from build123d import *

# Parameters (mm, degrees)
SKETCH2_R               = 21
SKETCH2_R_2             = 10.5
CUT_EXTRUDE1_DEPTH      = 11
CUT_EXTRUDE1_DEPTH_BACK = 12
SKETCH2_5_R             = 10.5
CUT_EXTRUDE2_DEPTH      = 12
CHAMFER1_SIZE           = 0.5


with BuildPart() as part:
    # Sketch1 → Revolve1 (revolve)
    with BuildSketch(Plane.XY):
        with BuildLine():
            Line((0, 10), (0, -11))
            Line((0, -11), (-21, -11))
            ThreePointArc((-21, -11), (-14.849242405, 3.849242405), (0, 10))
        make_face()
    revolve(axis=Axis((0, 10, 0), (0, -1, 0)))

    # Sketch2 → Cut-Extrude1 (cut, two sides)
    with BuildSketch(Plane(origin=(0, 0, 0), x_dir=(1, 0, 0), z_dir=(0, 1, 0))) as cut_extrude1_sk:
        Circle(SKETCH2_R)
        Circle(SKETCH2_R_2, mode=Mode.SUBTRACT)
    extrude(amount=CUT_EXTRUDE1_DEPTH, mode=Mode.SUBTRACT)
    extrude(cut_extrude1_sk.sketch, amount=-CUT_EXTRUDE1_DEPTH_BACK, mode=Mode.SUBTRACT)

    # Sketch2<5> → Cut-Extrude2 (cut, through all)
    with BuildSketch(Plane(origin=(0, 0, 0), x_dir=(1, 0, 0), z_dir=(0, 1, 0))):
        Circle(SKETCH2_5_R)
    extrude(amount=-CUT_EXTRUDE2_DEPTH, mode=Mode.SUBTRACT)

    # Chamfer1
    chamfer1_edges = [part.edges().sort_by_distance(p)[0] for p in [
        (-10.5, 0, 0),
    ]]
    chamfer(chamfer1_edges, length=CHAMFER1_SIZE)


solid = part.part
Read the model definition and answer for the solid it produces. Units are mm, in the model's axes. Coordinates: 2 decimals unless noted, no trailing zeros. Loops run counter-clockwise (first coordinate to the right, second up) from the corner with the lowest first, then second, coordinate; pieces in that order, holes last.
Q1. The part is cut by section C-C on y = 5. Write down the section's boundary in (x, z), and give its area (3 significant figures).
Q2. Each of these flat-tipped pins is pushed along its axis until it touches: pin 1 Ø6 at (x, y) = (8.5, 6) entering from +Z; pin 2 Ø5 at (y, z) = (2, 7) entering from -X; pin 3 Ø6 at (x, y) = (-5, 2.5) entering from -Z. Where does it stop, or does it pass through?
Q3. Consider probe 1 along Z at (x, y) = (-7, 4); probe 2 along X at (y, z) = (7, -1); probe 3 along Y at (x, z) = (9.25, -4.5). Determine where each line is inside the solid, lowest interval first.
Q4. The part is cut by section B-B on x = 0. Write down the section's boundary in (y, z).
Q5. The part is cut by section A-A on z = 0. Write down the section's boundary in (x, y).
Results below:
1. outline: circle Ø21 at (0, 0)
1. area: 346 mm2
2. pin 1: stops at z = 8.94
2. pin 2: stops at x = -9.49
2. pin 3: stops at z = -10.31
3. probe 1: z = -7.83 to 7.83
3. probe 2: x = -10.45 to 10.45
3. probe 3: y = 0.29 to 7.31
4. outline: (0, -10) - (0.5, -10.5) - (7.19, -10.5) arc R21 ccw to (7.19, 10.5) - (0.5, 10.5) - (0, 10) - close
5. outline: (-10.5, 0.5) - (-10, 0) - (10, 0) - (10.5, 0.5) - (10.5, 7.19) arc R21 ccw to (-10.5, 7.19) - close
